from build123d import *

# Parameters (mm, degrees)
SKETCH1_R           = 1.1
BOSS_EXTRUDE1_DEPTH = 7
CUT_EXTRUDE1_DEPTH  = 2.5


with BuildPart() as part:
    # Sketch1 → Boss-Extrude1 (new body)
    with BuildSketch(Plane.XY):
        with BuildLine():
            Line((3, 0), (17, 0))
            ThreePointArc((17, 0), (19.121320344, 0.878679656), (20, 3))
            Line((20, 3), (20, 5.5))
            Line((20, 5.5), (30, 5.5))
            ThreePointArc((30, 5.5), (32.121320344, 6.378679656), (33, 8.5))
            Line((33, 8.5), (33, 25.5))
            ThreePointArc((33, 25.5), (32.121320344, 27.621320344), (30, 28.5))
            Line((30, 28.5), (20.171059892, 28.5))
            ThreePointArc((20.171059892, 28.5), (19.080167127, 28.294629309), (18.138632628, 27.706635315))
            Line((18.138632628, 27.706635315), (0.967572736, 11.891185415))
            ThreePointArc((0.967572736, 11.891185415), (0.252520993, 10.889273762), (0, 9.684550099))
            Line((0, 9.684550099), (0, 3))
            ThreePointArc((0, 3), (0.878679656, 0.878679656), (3, 0))
        make_face()
        with Locations((5.2, 7)):
            Circle(SKETCH1_R, mode=Mode.SUBTRACT)
        with Locations((14.8, 7)):
            Circle(SKETCH1_R, mode=Mode.SUBTRACT)
        with BuildLine():
            Line((27.6, 21), (27.6, 13))
            ThreePointArc((27.6, 13), (25, 10.4), (22.4, 13))
            Line((22.4, 13), (22.4, 21))
            ThreePointArc((22.4, 21), (25, 23.6), (27.6, 21))
        make_face(mode=Mode.SUBTRACT)
    extrude(amount=BOSS_EXTRUDE1_DEPTH)

    # Sketch2 → Cut-Extrude1 (cut)
    with BuildSketch(Plane(origin=(0, 0, 0), x_dir=(-1, 0, 0), z_dir=(0, 0, -1))):
        with BuildLine():
            Line((-20.25, 21), (-20.25, 13))
            ThreePointArc((-20.25, 13), (-25, 8.25), (-29.75, 13))
            Line((-29.75, 13), (-29.75, 21))
            ThreePointArc((-29.75, 21), (-25, 25.75), (-20.25, 21))
        make_face()
    extrude(amount=-CUT_EXTRUDE1_DEPTH, mode=Mode.SUBTRACT)


solid = part.part
Geometry: final body of the model. Coordinates: model frame, mm. A direction names the side the tool comes from. Coordinates: 2 decimals unless noted, no trailing zeros. Order: outer loops, then holes, each group sorted by start corner. A loop starts at its lowest first (then second) coordinate and runs counter-clockwise, first axis right, second up. Notation, with made-up numbers: M 79,-10 L 117,-10 A17 cw 117,-1 Z; hole C -29.75,25 d8. An arc over 180 degrees is marked long. One line per question, with ' | ' between items. Start each with the question number.
Item 1: Pin query (flat end, axial travel): pin 1 Ø1.8 at (x, y) = (5.2, 7) entering from -Z; pin 2 Ø7.5 at (x, y) = (24.5, 14) entering from -Z; pin 3 Ø3.5 at (x, z) = (26, 4) entering from -Y; pin 4 Ø1.2 at (y, z) = (18.5, 1.5) entering from -X. Return the tip coordinate at first contact, or that it passes through.
Item 2: Cut plane D-D, the plane x = 14.8. Return the cut outline in (y, z), then the cut area to 3 significant figures.
Item 3: Draft query along X for faces 1 (the flat face through (16, 14, 7)), 2 (the cylindrical face through (0.86, 0.9, 3.45)), 3 (the cylindrical face through (19.1, 0.86, 3.45)), 4 (the cylindrical face through (24.9, 8.25, 1.23)). Return one class per face: released by +X, released by -X, zero draft, split by the parting line, or undercut.
Item 4: Ray query, probe 1 along X at (y, z) = (7.75, 6.5); probe 2 along X at (y, z) = (3, 1.75); probe 3 along X at (y, z) = (15.75, 3). Return the intervals inside material, ascending. Write a range as [from, to].
Item 5: Cut plane A-A, the plane z = 1. Return the cut outline in (x, y), then the cut area to 3 significant figures.
Item 6: Cut plane C-C, the plane y = 7. Return the cut outline in (x, z), then the cut area to 3 significant figures.
Item 7: Set-up query: faces 5 (the flat face through (29.75, 17, 1)), 6 (the flat face through (27.6, 17, 5)), 7 (the flat face through (20, 4, 3)). Return all of +Z, -Z, +X, -X, +Y, -Y with unobstructed straight access to the full face (end or side cutting, diameter ignored); none if empty.
Item 8: Cut plane B-B, the plane x = 25. Return the cut outline in (y, z).
A:
1) pin 1: passes through | pin 2: stops at z = 2.5 | pin 3: stops at y = 5.5 | pin 4: stops at x = 7.49
2) outline: M 0,0 L 5.9,0 L 5.9,7 L 0,7 Z; M 8.1,0 L 24.63,0 L 24.63,7 L 8.1,7 Z | area: 157 mm2
3) face 1: zero draft | face 2: released by -X | face 3: released by +X | face 4: undercut
4) probe 1: x = [0, 4.4], [6, 14], [15.6, 32.9] | probe 2: x = [0, 20] | probe 3: x = [5.16, 22.4], [27.6, 33]
5) outline: M 0,3 A3 ccw 3,0 L 17,0 A3 ccw 20,3 L 20,5.5 L 30,5.5 A3 ccw 33,8.5 L 33,25.5 A3 ccw 30,28.5 L 20.17,28.5 A3 ccw 18.14,27.71 L 0.97,11.89 A3 ccw 0,9.68 Z; hole C 5.2,7 d2.2; hole C 14.8,7 d2.2; hole M 20.25,13 A4.75 ccw 29.75,13 L 29.75,21 A4.75 ccw 20.25,21 Z | area: 540 mm2
6) outline: M 0,0 L 4.1,0 L 4.1,7 L 0,7 Z; M 6.3,0 L 13.7,0 L 13.7,7 L 6.3,7 Z; M 15.9,0 L 32.6,0 L 32.6,7 L 15.9,7 Z | area: 197 mm2
7) face 5: -Z | face 6: +Z, -Z | face 7: +Z, -Z, +X, -Y
8) outline: M 5.5,0 L 8.25,0 L 8.25,2.5 L 10.4,2.5 L 10.4,7 L 5.5,7 Z; M 23.6,2.5 L 25.75,2.5 L 25.75,0 L 28.5,0 L 28.5,7 L 23.6,7 Z
